Check sheet for the modelled part. Datum: model origin and axes. Units: mm. Face numbers are marked on the shaded views. A direction names the side the tool comes from. Give positions to 0.01 mm unless a question says otherwise; leave off trailing zeros. Write each loop counter-clockwise with the first axis right and the second up, starting at its lowest first coordinate (ties: lowest second). Pieces come first, ordered by that corner, then holes. Notation, with made-up numbers: M 48,-14.75 L 52,-14.75 A22 cw 52,22.25 Z; hole C -11,32 d9. An arc over 180 degrees is marked long. Use CSV: the item, a comma, the result in double quotes. Start each with the question number.
1. Depth check by flat-ended pin: P1, Ø7.5, axis at x = 23.5, y = -12, coming from the +Z side; P2, Ø6, axis at x = 15, z = 20, coming from the +Y side. Enter the tip coordinate at first touch or a pass-through.
2. Access from +Z, -Z, +X, -X, +Y, -Y to the whole of each face (thin tool, end or side, straight path). Record for the marked faces 1 and 2.
3. Scan lines: line 1 (Z direction, x = 41, y = -15.5); line 2 (X direction, y = -15, z = 14); line 3 (Y direction, x = 27, z = 19.25). Record each from-to range of solid material in increasing order.
4. Cross-section at A-A, the plane z = 19. Enter the section's corners in (x, y).
5. Cross-section at D-D, the plane x = 10. Enter the section's corners in (y, z), and give its area (3 significant figures).
6. Cross-section at C-C, the plane x = 27. Enter the section's corners in (y, z).
7. Mould release check, pull along Y, two halves, no side actions. Record for the marked faces 3, 4 and 5: +Y half, -Y half, draft (parallel to the pull), parting line (faces both ways), or undercut.
8. Cross-section at B-B, the plane y = -15.75. Enter the section's corners in (x, z).
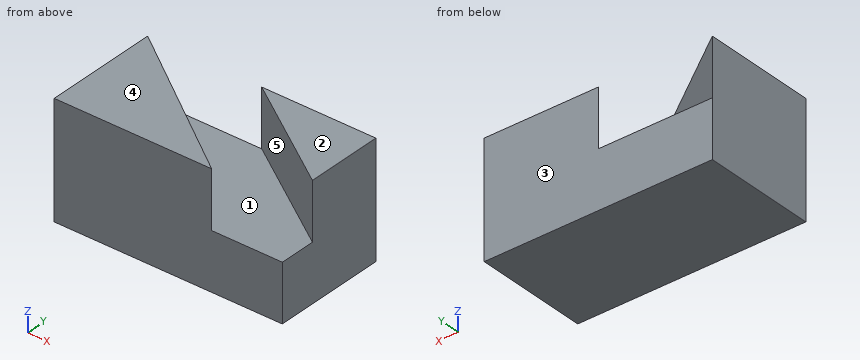
from build123d import *

# Parameters (mm, degrees)
F0_W     = 12.7
F0_H     = 12.7
F1_DEPTH = 25.4
F3_DEPTH = 12.7


with BuildPart() as f1:
    # F0 (on Front) → F1 (new body)
    with BuildSketch(Plane.XZ):
        Polygon((0, 25.4), (0, 0), (50.8, 0), (50.8, 12.7), (38.1, 12.7), (38.1, 25.4), align=None)
        with Locations((44.45, 19.05)):
            Rectangle(F0_W, F0_H)
    extrude(amount=F1_DEPTH)

    # F2 (on face) → F3 (cut, symmetric)
    with BuildSketch(Plane.XY.offset(25.4)):
        Polygon((25.4, 0), (0, 0), (35.067357, -25.4), (50.8, -25.4), (50.8, -17.231373), align=None)
    extrude(amount=F3_DEPTH, both=True, mode=Mode.SUBTRACT)


solid = f1.part
Worked answers:
1,P1,"stops at z = 12.7"
1,P2,"stops at y = -8.69"
2,face 1,"+Z"
2,face 2,"+Z, +X, -X, +Y, -Y"
3,line 1,"z = 0 to 12.7"
3,line 2,"x = 0 to 20.71, 47.51 to 50.8"
3,line 3,"y = -25.4 to -19.56, -1.09 to 0"
4,outline,"M 0,-25.4 L 35.07,-25.4 L 0,0 Z; M 25.4,0 L 50.8,-17.23 L 50.8,0 Z"
5,outline,"M -25.4,0 L 0,0 L 0,12.7 L -7.24,12.7 L -7.24,25.4 L -25.4,25.4 Z"
5,area,"553 mm^2"
6,outline,"M -25.4,0 L 0,0 L 0,25.4 L -1.09,25.4 L -1.09,12.7 L -19.56,12.7 L -19.56,25.4 L -25.4,25.4 Z"
7,face 3,"+Y half"
7,face 4,"draft"
7,face 5,"undercut"
8,outline,"M 0,0 L 50.8,0 L 50.8,25.4 L 48.62,25.4 L 48.62,12.7 L 21.74,12.7 L 21.74,25.4 L 0,25.4 Z"
